Check sheet for the drawn part. Datum: minimum x, y, z corner. Units: mm. Give positions to 0.01 mm unless a question says otherwise; leave off trailing zeros. Write each loop counter-clockwise with the first axis right and the second up, starting at its lowest first coordinate (ties: lowest second). Pieces come first, ordered by that corner, then holes. Notation, with made-up numbers: M -34,-11 L 19,-11 A11 ccw 19,2 Z; hole C 60,81.5 d10. An arc over 180 degrees is marked long. Use CSV: the item, a comma, the result in double quotes. Start each with the question number.
1. Mould release check, pull along X, two halves, no side actions. Record for the marked faces 1 and 2: +X half, -X half, draft (parallel to the pull), parting line (faces both ways), or undercut.
2. Depth check by flat-ended pin: P1, Ø1, axis at y = 82.5, z = 151.5, coming from the -X side; P2, Ø0.9, axis at y = 115, z = 173, coming from the -X side; P3, Ø0.9, axis at y = 115, z = 96.5, coming from the +X side. Enter the tip coordinate at first touch or a pass-through.
3. Cross-section at A-A, the plane z = 126.5. Enter the section's corners in (x, y), and give its area (3 significant figures).
4. Scan lines: line 1 (Y direction, x = 88, z = 144.5); line 2 (X direction, y = 90.5, z = 79); line 3 (X direction, y = 10, z = 111). Record each from-to range of solid material in increasing order.
5. Cross-section at D-D, the plane y = 87. Enter the section's corners in (x, z).
6. Cross-section at B-B, the plane y = 60. Enter the section's corners in (x, z).
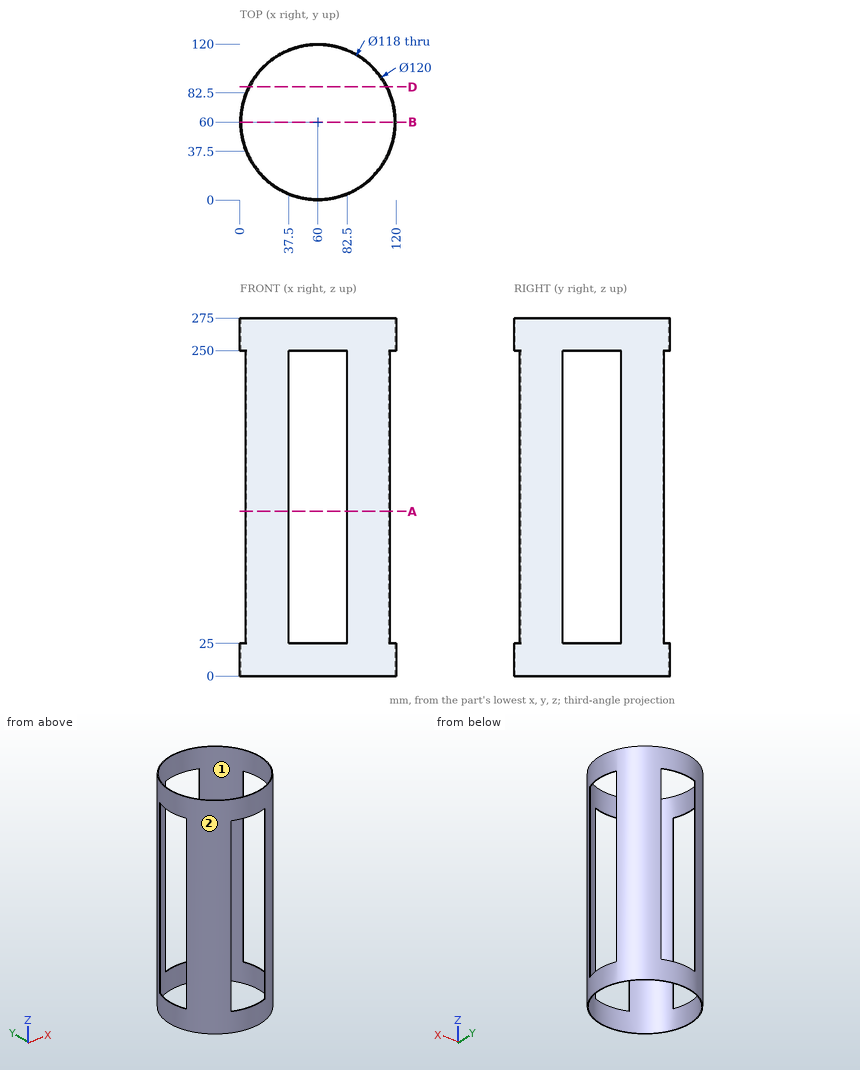
Worked answers:
1,face 1,"undercut"
1,face 2,"parting line"
2,P1,"stops at x = 4.38"
2,P2,"stops at x = 35.01"
2,P3,"stops at x = 84.99"
3,outline,"M 4.38,37.5 A60 ccw 37.5,4.38 L 37.5,5.46 A59 cw 5.46,37.5 Z; M 4.38,82.5 L 5.46,82.5 A59 cw 37.5,114.54 L 37.5,115.62 A60 ccw Z; M 82.5,4.38 A60 ccw 115.62,37.5 L 114.54,37.5 A59 cw 82.5,5.46 Z; M 82.5,114.54 A59 cw 114.54,82.5 L 115.62,82.5 A60 ccw 82.5,115.62 Z"
3,area,"189 mm^2"
4,line 1,"y = 6.93 to 8.07, 111.93 to 113.07"
4,line 2,"x = 8.33 to 9.5, 110.5 to 111.67"
4,line 3,"x = 26.83 to 28.68, 91.32 to 93.17"
5,outline,"M 6.42,0 L 7.54,0 L 7.54,275 L 6.42,275 Z; M 112.46,0 L 113.58,0 L 113.58,275 L 112.46,275 Z"
6,outline,"M 0,0 L 1,0 L 1,25 L 0,25 Z; M 0,250 L 1,250 L 1,275 L 0,275 Z; M 119,0 L 120,0 L 120,25 L 119,25 Z; M 119,250 L 120,250 L 120,275 L 119,275 Z"
